```python
from build123d import *

# Parameters (mm, degrees)
CROQUIS1_R              = 2.5
SALIENTE_EXTRUIR1_DEPTH = 12
CROQUIS2_R              = 5
SALIENTE_EXTRUIR2_DEPTH = 3
CROQUIS3_W              = 1.4
CROQUIS3_H              = 11
CORTAR_EXTRUIR2_DEPTH   = 2.5
CORTAR_EXTRUIR2_TAPER   = 9


with BuildPart() as part:
    # Croquis1 → Saliente-Extruir1 (new body)
    with BuildSketch(Plane.XY):
        Circle(CROQUIS1_R)
    extrude(amount=SALIENTE_EXTRUIR1_DEPTH)

    # Croquis2 → Saliente-Extruir2 (add)
    with BuildSketch(Plane.XY):
        Circle(CROQUIS2_R)
    extrude(amount=-SALIENTE_EXTRUIR2_DEPTH)

    # Croquis3 → Cortar-Extruir2 (cut)
    with BuildSketch(Plane(origin=(0, 0, -3), x_dir=(-1, 0, 0), z_dir=(0, 0, -1))):
        Rectangle(CROQUIS3_W, CROQUIS3_H)
    extrude(amount=-CORTAR_EXTRUIR2_DEPTH, taper=CORTAR_EXTRUIR2_TAPER, mode=Mode.SUBTRACT)


solid = part.part
```
Could you check a few things on this model? Use its own coordinates, in mm. A direction names the side the tool comes from. Coordinates: 2 decimals unless noted, no trailing zeros. Loops run counter-clockwise (first coordinate to the right, second up) from the corner with the lowest first, then second, coordinate; pieces in that order, holes last.
1) Which directions (+Z, -Z, +X, -X, +Y, -Y) give clear straight access to the entire face, cutting with the end or side of a thin tool? Please do faces 1 (the face through (2, 0, -3)), 2 (the face through (2, -2, 0)).
Reported:
face 1: -Z, +X, -X, +Y, -Y
face 2: +Z
2) Imagine slicing it at A-A (x = 0). List the corners of the cut face in (y, z) for me, and give its area (3 significant figures).
Reported:
outline: (-5, -0.5) - (5, -0.5) - (5, 0) - (2.5, 0) - (2.5, 12) - (-2.5, 12) - (-2.5, 0) - (-5, 0) - close
area: 65.0 mm2
3) Will these pins go through, and if not, where does the flat tip stop? pin 1 Ø1 at (x, z) = (0.5, 8) entering from -Y; pin 2 Ø1.5 at (x, z) = (-3.5, -1) entering from +Y; pin 3 Ø3 at (y, z) = (3.5, 6.5) entering from -X.
Reported:
pin 1: stops at y = -2.5
pin 2: stops at y = 4.18
pin 3: stops at x = -1.5
4) Please list where these lines run through material, in increasing order: line 1 along Y through (x, z) = (0, 8); line 2 along Z through (x, y) = (-3.75, 0.5); line 3 along X through (y, z) = (-2, -1.25).
Reported:
line 1: y = -2.5 to 2.5
line 2: z = -3 to 0
line 3: x = -4.58 to -0.42, 0.42 to 4.58
5) Imagine slicing it at C-C (x = 1.25). List the corners of the cut face in (y, z) for me.
Reported:
outline: (-4.84, -3) - (4.84, -3) - (4.84, 0) - (2.17, 0) - (2.17, 12) - (-2.17, 12) - (-2.17, 0) - (-4.84, 0) - close
6) Imagine slicing it at B-B (z = 3.5). List the corners of the cut face in (x, y) for me.
Reported:
outline: circle Ø5 at (0, 0)
7) Imagine slicing it at D-D (x = 3.25). List the corners of the cut face in (y, z) for me, and give its area (3 significant figures).
Reported:
outline: (-3.8, -3) - (3.8, -3) - (3.8, 0) - (-3.8, 0) - close
area: 22.8 mm2
